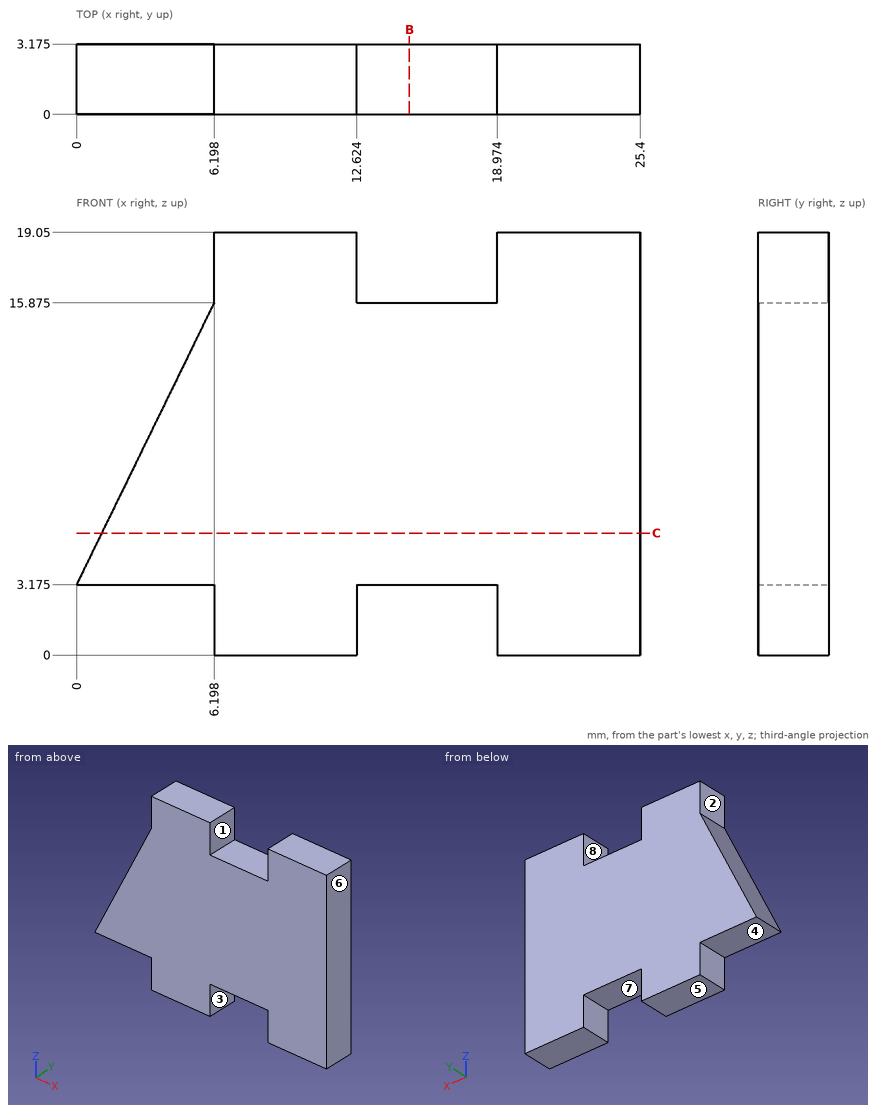
Here's the drawing with two shaded views (mm, measured from the low corner). I have some questions. A direction names the side the tool comes from. Give positions to 0.01 mm unless a question says otherwise; leave off trailing zeros. Write each loop counter-clockwise with the first axis right and the second up, starting at its lowest first coordinate (ties: lowest second). Pieces come first, ordered by that corner, then holes. Notation, with made-up numbers: (-20.5, 59.5) -> (24.5, 59.5) arc R31 cw to (24.5, 83.5) -> close; hole circle Ø11 at (-12.5, -34). An arc over 180 degrees is marked (long way). One line per item, written item: value.
Q1. Imagine slicing it at B-B on x = 15. Please give me the cut outline in (y, z) (1 decimal), and give its area (3 significant figures).
Results found:
outline: (0, 3.2) -> (3.2, 3.2) -> (3.2, 15.9) -> (0, 15.9) -> close
area: 40.3 mm^2
Q2. We'd pull the mould along X, two halves only. Please class the marked faces 5, 6, 7 and 8: +X half, -X half, draft (parallel to the pull), parting line (faces both ways), or undercut.
Results found:
face 5: draft
face 6: +X half
face 7: undercut
face 8: undercut
Q3. For P1, Ø1.6, axis at x = 4.5, y = 2, coming from the -Z side (3 decimals); P2, Ø1.6, axis at x = 17.5, y = 2.5, coming from the +Z side (3 decimals); P3, Ø1, axis at y = 1, z = 6.5, coming from the -X side, each with a flat end and sliding along its axis, tell me the tip position at first contact or that it passes through.
Results found:
P1: stops at z = 3.175
P2: stops at z = 15.875
P3: stops at x = 1.38
Q4. Which directions (+Z, -Z, +X, -X, +Y, -Y) give clear straight access to the entire face, cutting with the end or side of a thin tool? Please do the marked faces 1, 2, 3 and 4.
Results found:
face 1: +Z, +Y, -Y
face 2: +Z, -X, +Y, -Y
face 3: -Z, +Y, -Y
face 4: -Z, -X, +Y, -Y
Q5. Imagine slicing it at C-C on z = 5.5. Please give me the cut outline in (x, y) (1 decimal).
Results found:
outline: (1.1, 0) -> (25.4, 0) -> (25.4, 3.2) -> (1.1, 3.2) -> close
Q6. Please list where these lines run through material, in increasing order: line 1 (X direction, y = 2.7, z = 3); line 2 (Z direction, x = 14.5, y = 0.6) (1 decimal); line 3 (Z direction, x = 3.75, y = 1.5) (1 decimal). Write a range as [from, to].
Results found:
line 1: x = [6.2, 12.62], [18.97, 25.4]
line 2: z = [3.2, 15.9]
line 3: z = [3.2, 10.9]
